CAD build for the part. Positions are in the model's coordinates, mm. Face numbers are marked on the shaded views. A direction names the side the tool comes from. Give positions to 0.01 mm unless a question says otherwise; leave off trailing zeros. Loops run counter-clockwise (first coordinate to the right, second up) from the corner with the lowest first, then second, coordinate; pieces in that order, holes last. Notation, with made-up numbers: (62.5, 8.25) -> (118.5, 8.25) arc R17 ccw to (118.5, 35.25) -> close; hole circle Ø1 at (-30, 54). An arc over 180 degrees is marked (long way). Use one line per item in the form item = value.
Autodesk Inventor part; units mm, degrees
ref_plane "YZ Plane" through (0, 0, 0) normal (1, 0, 0) x (0, 1, 0)
ref_plane "XZ Plane" through (0, 0, 0) normal (0, 1, 0) x (-1, 0, 0)
ref_plane "XY Plane" through (0, 0, 0) normal (0, 0, 1) x (1, 0, 0)
sketch "Sketch1" plane through (0, 0, 0) normal (0, 0, 1) x (1, 0, 0)
  line L0 (6.9242, 30.3294) -> (37.9242, 30.3294)
  line L1 (37.9242, 30.3294) -> (37.9242, 12.3294)
  line L2 (37.9242, 12.3294) -> (6.9242, 12.3294)
  line L3 (6.9242, 12.3294) -> (6.9242, 30.3294)
  point P0 (0, 0)
  dimension "d0" = 31
  dimension "d1" = 18
extrude "Extrusion1" add sketch "Sketch1" along normal blind 1.5
sketch "Sketch2" plane through (0, 0, 1.5) normal (0, 0, 1) x (1, 0, 0)
  line L0 (37.9242, 30.3294) -> (6.9242, 30.3294)
  line L1 (6.9242, 30.3294) -> (9.9242, 30.3294)
  line L2 (9.9242, 30.3294) -> (9.9242, 12.3294)
  line L3 (9.9242, 12.3294) -> (6.9242, 12.3294)
  line L4 (6.9242, 12.3294) -> (6.9242, 30.3294)
  line L5 (37.9242, 12.3294) -> (37.9242, 30.3294)
  line L6 (37.9242, 30.3294) -> (34.9242, 30.3294)
  line L7 (34.9242, 30.3294) -> (34.9242, 12.3294)
  line L8 (34.9242, 12.3294) -> (37.9242, 12.3294)
  line L9 (37.9242, 12.3294) -> (37.9242, 30.3294)
  point P0 (0, 0)
  dimension "d4" = 3
  dimension "d5" = 18
  dimension "d6" = 3
  dimension "d7" = 18
extrude "Extrusion2" add sketch "Sketch2" along normal blind 13
sketch "Sketch3" plane through (6.9242, 12.3294, 0) normal (-1, 0, 0) x (0, 0, 1)
  line L0 (0, 18) -> (0, 0)
  circle A0 centre (7, 9) radius 2.5
  point P0 (0, -12.3294)
extrude "Extrusion3" cut sketch "Sketch3" against normal blind 50
sketch "Sketch4" plane through (0, 0, 1.5) normal (0, 0, 1) x (1, 0, 0)
  line L0 (37.9242, 30.3294) -> (6.9242, 30.3294)
  line L1 (6.9242, 12.3294) -> (37.9242, 12.3294)
  circle A0 centre (22.4242, 21.3294) radius 2.5
  point P0 (0, 0)
extrude "Extrusion4" cut sketch "Sketch4" against normal blind 50
thread "Thread1"
thread "Thread2"
thread "Thread3"
properties part number "penyangga kamera 1"
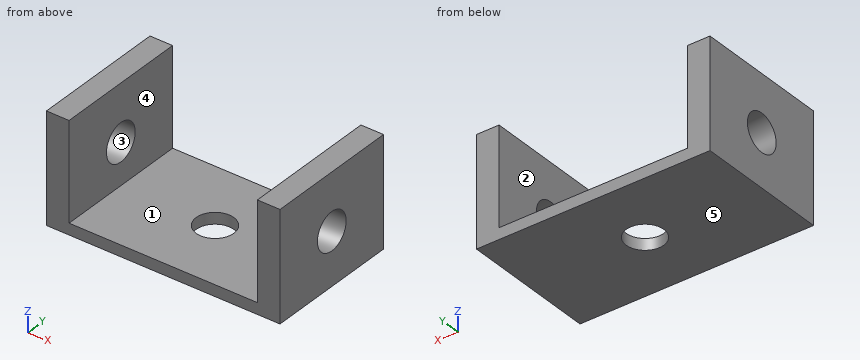
1. Cut at B-B, the plane z = 7. Write the cut outline in (x, y), then the cut area to 3 significant figures.
Result sheet:
outline = (6.92, 12.33) -> (9.92, 12.33) -> (9.92, 18.83) -> (6.92, 18.83) -> close; (6.92, 23.83) -> (9.92, 23.83) -> (9.92, 30.33) -> (6.92, 30.33) -> close; (34.92, 12.33) -> (37.92, 12.33) -> (37.92, 18.83) -> (34.92, 18.83) -> close; (34.92, 23.83) -> (37.92, 23.83) -> (37.92, 30.33) -> (34.92, 30.33) -> close
area = 78.0 mm^2
2. Drill centre lines: line 1 (X direction, y = 21.75, z = 14.25); line 2 (Y direction, x = 37.3, z = 7); line 3 (Z direction, x = 10.5, y = 15.25). Where is each one in solid material? Low to high.
Result sheet:
line_1 = 6.92 to 9.92, 34.92 to 37.92
line_2 = 12.33 to 18.83, 23.83 to 30.33
line_3 = 0 to 1.5
3. Mould opens along Z. For the marked faces 1, 2 and 3 say: pulls with the +Z half, pulls with the -Z half, needs draft (parallel to the pull), parting line crosses it, or undercut.
Result sheet:
face_1 = pulls with the +Z half
face_2 = needs draft
face_3 = undercut
4. Cut at D-D, the plane y = 28.5. Write the cut outline in (x, z), then the cut area to 4 significant figures.
Result sheet:
outline = (6.92, 0) -> (37.92, 0) -> (37.92, 14.5) -> (34.92, 14.5) -> (34.92, 1.5) -> (9.92, 1.5) -> (9.92, 14.5) -> (6.92, 14.5) -> close
area = 124.5 mm^2
5. Drop a flat-ended pin along its axis: P1, Ø9, axis at x = 26.5, y = 18.5, coming from the +Z side. Give the stop position or say it passes through.
Result sheet:
P1 = 1.5
6. Cut at A-A, the plane z = 2.5. Write the cut outline in (x, y).
Result sheet:
outline = (6.92, 12.33) -> (9.92, 12.33) -> (9.92, 30.33) -> (6.92, 30.33) -> close; (34.92, 12.33) -> (37.92, 12.33) -> (37.92, 30.33) -> (34.92, 30.33) -> close
7. Cut at C-C, the plane x = 24.5. Write the cut outline in (y, z), then the cut area to 3 significant figures.
Result sheet:
outline = (12.33, 0) -> (19.94, 0) -> (19.94, 1.5) -> (12.33, 1.5) -> close; (22.72, 0) -> (30.33, 0) -> (30.33, 1.5) -> (22.72, 1.5) -> close
area = 22.8 mm^2
8. Tool access for the marked faces 4 and 5: list every direction of +Z, -Z, +X, -X, +Y, -Y with a clear straight run to the whole face (end or side of a thin tool).
Result sheet:
face_4 = +Z, +Y, -Y
face_5 = -Z, +X, -X, +Y, -Y
